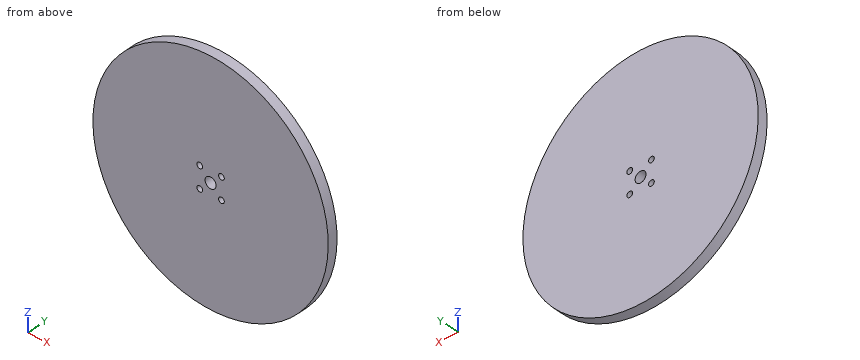
```python
from build123d import *

# Parameters (mm, degrees)
ESQUISSE1_R             = 75
BOSS_EXTRU_1_DEPTH      = 6.35
ESQUISSE2_R             = 3.5
ENL_V_MAT_EXTRU_1_DEPTH = 6.35
SKETCH1_R               = 1.8288
CUT_EXTRUDE1_DEPTH      = 6.35
CIRPATTERN1_COUNT       = 4


with BuildPart() as part:
    # Esquisse1 → Boss.-Extru.1 (new body)
    with BuildSketch(Plane(origin=(0, 0, 0), x_dir=(1, 0, 0), z_dir=(0, 1, 0))):
        with Locations(Location((0, 0, 0), (0, 0, 270))):
            Circle(ESQUISSE1_R)
    extrude(amount=BOSS_EXTRU_1_DEPTH)

    # Esquisse2 → Enlèv. mat.-Extru.1 (cut)
    with BuildSketch(Plane(origin=(0, 6.35, 0), x_dir=(1, 0, 0), z_dir=(0, 1, 0))):
        with Locations(Location((0, 0, 0), (0, 0, 270))):
            Circle(ESQUISSE2_R)
    extrude(amount=-ENL_V_MAT_EXTRU_1_DEPTH, mode=Mode.SUBTRACT)

    # Sketch1 → Cut-Extrude1 (cut)
    with BuildSketch(Plane.XZ):
        with Locations(Location((-6.914797213, 6.914797213, 0), (0, 0, 270))):
            Circle(SKETCH1_R)
    cut_extrude1 = extrude(amount=-CUT_EXTRUDE1_DEPTH, mode=Mode.SUBTRACT)

    # CirPattern1: Cut-Extrude1 ×4 about axis
    cirpattern1_axis = Axis((0, 0, 0), (0, 1, 0))
    for i in range(1, CIRPATTERN1_COUNT):
        add(cut_extrude1.rotate(cirpattern1_axis, i * 360 / CIRPATTERN1_COUNT), mode=Mode.SUBTRACT)


solid = part.part
```
Geometry: final body of the model. Coordinates: model frame, mm. Give positions to 0.01 mm unless a question says otherwise; leave off trailing zeros. Order: outer loops, then holes, each group sorted by start corner. A loop starts at its lowest first (then second) coordinate and runs counter-clockwise, first axis right, second up. Notation, with made-up numbers: (-22, 64) -> (35, 64) arc R16 ccw to (35, 89) -> close; hole circle Ø2 at (19.25, -24). An arc over 180 degrees is marked (long way). Write each question's results on one line, items separated by ' | '. Start each with the question number.
1) Section D-D (x = -51). Return loops of the section in (y, z).
2) Section C-C (y = 3.75). Return loops of the section in (x, z).
3) Line query: line 1 (X direction, y = 2.25, z = 0); line 2 (X direction, y = 1.25, z = -17); line 3 (X direction, y = 1.25, z = -59.5). Output: solid intervals per line, ascending. Write a range as from..to.
4) First-contact query: pin 1 (2 mm diameter, centred on x = 6.91, z = -6.91, fed in from -Y); pin 2 (3 mm diameter, centred on x = 20.5, y = 2.5, fed in from +Z); pin 3 (2 mm diameter, centred on x = 22, y = 1.5, fed in from -Z); pin 4 (3 mm diameter, centred on y = 1, z = 2.5, fed in from -X). Flat tips, straight axial feed; report the tip coordinate or a pass-through.
5) Section A-A (x = 0). Return loops of the section in (y, z).
6) Section B-B (z = 0). Return loops of the section in (x, y), then the cut area to 3 significant figures.
Calculated:
1) outline: (0, -54.99) -> (6.35, -54.99) -> (6.35, 54.99) -> (0, 54.99) -> close
2) outline: circle Ø150 at (0, 0); hole circle Ø3.66 at (-6.91, -6.91); hole circle Ø3.66 at (-6.91, 6.91); hole circle Ø7 at (0, 0); hole circle Ø3.66 at (6.91, -6.91); hole circle Ø3.66 at (6.91, 6.91)
3) line 1: -75..-3.5, 3.5..75 | line 2: -73.05..73.05 | line 3: -45.66..45.66
4) pin 1: through | pin 2: z = 72.55 | pin 3: z = -72 | pin 4: x = -74.99
5) outline: (0, -75) -> (6.35, -75) -> (6.35, -3.5) -> (0, -3.5) -> close; (0, 3.5) -> (6.35, 3.5) -> (6.35, 75) -> (0, 75) -> close
6) outline: (-75, 0) -> (-3.5, 0) -> (-3.5, 6.35) -> (-75, 6.35) -> close; (3.5, 0) -> (75, 0) -> (75, 6.35) -> (3.5, 6.35) -> close | area: 908 mm2
